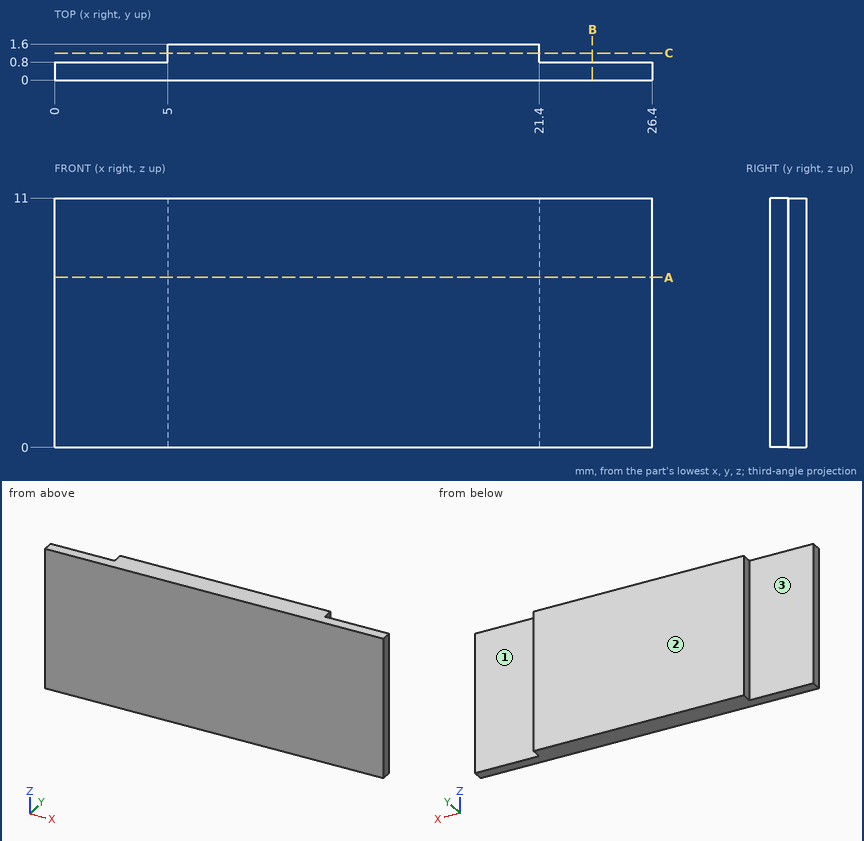
Check sheet for the drawn part. Datum: minimum x, y, z corner. Units: mm. A direction names the side the tool comes from. Give positions to 0.01 mm unless a question says otherwise; leave off trailing zeros. Write each loop counter-clockwise with the first axis right and the second up, starting at its lowest first coordinate (ties: lowest second). Pieces come first, ordered by that corner, then holes. Notation, with made-up numbers: (24, -28) -> (61, -28) arc R26 ccw to (61, -13) -> close; hole circle Ø7 at (83, 52). An arc over 180 degrees is marked (long way). Use one line per item in the form item = value. Start each with the question number.
1. Section check B-B (x = 23.75). Record the cut outline in (y, z).
2. Section check C-C (y = 1.2). Record the cut outline in (x, z), and give its area (3 significant figures).
3. Thickness scan on line 1 along X through (y, z) = (1.1, 5.5); line 2 along Y through (x, z) = (3.75, 7). Record the ranges inside material, lowest first. Write a range as from..to.
4. Access from +Z, -Z, +X, -X, +Y, -Y to the whole of each face (thin tool, end or side, straight path). Record for the marked faces 1, 2 and 3.
5. Section check A-A (z = 7.5). Record the cut outline in (x, y).
6. Go/stop test with flat-tipped pins: P1, Ø5.5, axis at x = 1.5, z = 6, coming from the +Y side; P2, Ø0.6, axis at y = 1.5, z = 3, coming from the -X side. Record where each tip stops, or that it passes through.
Conclusion:
q1.outline = (0, 0) -> (0.8, 0) -> (0.8, 11) -> (0, 11) -> close
q2.outline = (5, 0) -> (21.4, 0) -> (21.4, 11) -> (5, 11) -> close
q2.area = 180 mm²
q3.line_1 = 5..21.4
q3.line_2 = 0..0.8
q4.face_1 = +Z, -Z, +X, +Y
q4.face_2 = +Z, -Z, +X, -X, +Y
q4.face_3 = +Z, -Z, -X, +Y
q5.outline = (0, 0) -> (26.4, 0) -> (26.4, 0.8) -> (21.4, 0.8) -> (21.4, 1.6) -> (5, 1.6) -> (5, 0.8) -> (0, 0.8) -> close
q6.P1 = 0.8
q6.P2 = 5
